Source: CAD feature listing. Evaluate the final solid. Frame: model axes, mm. Round coordinates to 2 decimals unless told otherwise and drop trailing zeros. Order: outer loops, then holes, each group sorted by start corner. A loop starts at its lowest first (then second) coordinate and runs counter-clockwise, first axis right, second up. Notation, with made-up numbers: (-35, 43) -> (4, 43) arc R8 ccw to (4, 57) -> close; hole circle Ø1 at (-19, -17.75). An arc over 180 degrees is marked (long way). Write item = value, one per line. Start each with the question number.
(1) Cut plane A-A on x = 14. Return the cut outline in (y, z) (3 decimals).
(2) Contact query for flat-ended pins moving along their axis: pin 1 Ø2 at (y, z) = (-6, -2.5) entering from +X; pin 2 Ø12 at (y, z) = (-13.5, 16.5) entering from +X; pin 3 Ø3 at (x, y) = (1.5, -11.5) entering from -Z. Output: stop coordinate, or through.
(3) Cut plane B-B on z = 19. Return the cut outline in (x, y), then the cut area to 3 significant figures.
(4) Ray query, line 1 (X direction, y = -10, z = 0); line 2 (Z direction, x = -9.5, y = -7); line 3 (Z direction, x = 12, y = -32). Return the intervals inside material, ascending.
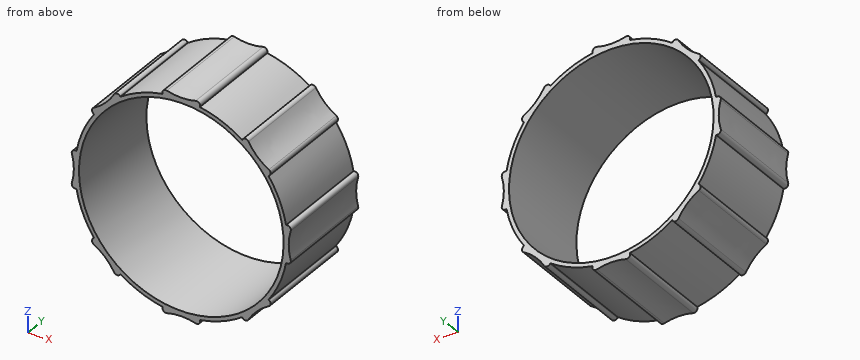
from build123d import *

# Parameters (mm, degrees)
SKETCH3_R           = 37.8587
BOSS_EXTRUDE1_DEPTH = 37.5666


with BuildPart() as part:
    # Sketch3 → Boss-Extrude1 (new body)
    with BuildSketch(Plane(origin=(0, -37.5666, 0), x_dir=(1, 0, 0), z_dir=(0, 1, 0))):
        with BuildLine():
            Line((22.710713351, 32.518210948), (22.542535263, 32.277406051))
            ThreePointArc((22.542535263, 32.277406051), (15.06624702, 36.373135768), (6.883594535, 38.763551242))
            Line((6.883594535, 38.763551242), (6.934949387, 39.052745559))
            ThreePointArc((6.934949387, 39.052745559), (6.539953295, 40.213477214), (5.347634612, 40.499302411))
            add(Edge.make_bspline(
                [(5.347634612, 40.499302411), (0, 39.028097589), (-5.347634612, 40.499302411)],
                knots=[0.133971893, 0.133971893, 0.133971893, 0.866028107, 0.866028107, 0.866028107], degree=2))
            ThreePointArc((-5.347634612, 40.499302411), (-6.539953295, 40.213477214), (-6.934949387, 39.052745559))
            Line((-6.934949387, 39.052745559), (-6.883594478, 38.763550918))
            ThreePointArc((-6.883594478, 38.763550918), (-15.06624685, 36.373135059), (-22.542534901, 32.277404991))
            Line((-22.542534901, 32.277404991), (-22.7107128, 32.518209618))
            ThreePointArc((-22.7107128, 32.518209618), (-23.810778439, 33.059666427), (-24.855984001, 32.418678735))
            add(Edge.make_bspline(
                [(-24.855984001, 32.418678735), (-27.597033743, 27.597031182), (-32.418681395, 24.855981341)],
                knots=[0.133971893, 0.133971893, 0.133971893, 0.866028107, 0.866028107, 0.866028107], degree=2))
            ThreePointArc((-32.418681395, 24.855981341), (-33.059669087, 23.810775779), (-32.518212278, 22.71071014))
            Line((-32.518212278, 22.71071014), (-32.277407381, 22.542532053))
            ThreePointArc((-32.277407381, 22.542532053), (-36.373137098, 15.066243809), (-38.763552571, 6.883591325))
            Line((-38.763552571, 6.883591325), (-39.052746889, 6.934946176))
            ThreePointArc((-39.052746889, 6.934946176), (-40.213478544, 6.539950084), (-40.499303741, 5.347631401))
            add(Edge.make_bspline(
                [(-40.499303741, 5.347631401), (-39.028096259, -3.092e-06), (-40.499303741, -5.347637823)],
                knots=[0.133971893, 0.133971893, 0.133971893, 0.866028107, 0.866028107, 0.866028107], degree=2))
            ThreePointArc((-40.499303741, -5.347637823), (-40.213478544, -6.539956506), (-39.052746889, -6.934952598))
            Line((-39.052746889, -6.934952598), (-38.763552248, -6.883597689))
            ThreePointArc((-38.763552248, -6.883597689), (-36.373136389, -15.066250061), (-32.277406321, -22.542538112))
            Line((-32.277406321, -22.542538112), (-32.518210948, -22.710716011))
            ThreePointArc((-32.518210948, -22.710716011), (-33.059667757, -23.81078165), (-32.418680065, -24.855987212))
            add(Edge.make_bspline(
                [(-32.418680065, -24.855987212), (-27.597028006, -27.597032378), (-24.855982671, -32.418684606)],
                knots=[0.133971893, 0.133971893, 0.133971893, 0.866028107, 0.866028107, 0.866028107], degree=2))
            ThreePointArc((-24.855982671, -32.418684606), (-23.810777109, -33.059672297), (-22.71071147, -32.518215489))
            Line((-22.71071147, -32.518215489), (-22.542533383, -32.277410592))
            ThreePointArc((-22.542533383, -32.277410592), (-15.066245139, -36.373140308), (-6.883592655, -38.763555782))
            Line((-6.883592655, -38.763555782), (-6.934947506, -39.0527501))
            ThreePointArc((-6.934947506, -39.0527501), (-6.539951414, -40.213481755), (-5.347632731, -40.499306952))
            add(Edge.make_bspline(
                [(-5.347632731, -40.499306952), (1.811e-06, -39.028093048), (5.347636493, -40.499306952)],
                knots=[0.133971893, 0.133971893, 0.133971893, 0.866028107, 0.866028107, 0.866028107], degree=2))
            ThreePointArc((5.347636493, -40.499306952), (6.539955176, -40.213481755), (6.934951268, -39.0527501))
            Line((6.934951268, -39.0527501), (6.883596359, -38.763555459))
            ThreePointArc((6.883596359, -38.763555459), (15.066248731, -36.3731396), (22.542536782, -32.277409531))
            Line((22.542536782, -32.277409531), (22.710714681, -32.518214159))
            ThreePointArc((22.710714681, -32.518214159), (23.81078032, -33.059670967), (24.855985882, -32.418683276))
            add(Edge.make_bspline(
                [(24.855985882, -32.418683276), (27.597029251, -27.597029251), (32.418683276, -24.855985882)],
                knots=[0.133971893, 0.133971893, 0.133971893, 0.866028107, 0.866028107, 0.866028107], degree=2))
            ThreePointArc((32.418683276, -24.855985882), (33.059670967, -23.81078032), (32.518214159, -22.710714681))
            Line((32.518214159, -22.710714681), (32.277409262, -22.542536593))
            ThreePointArc((32.277409262, -22.542536593), (36.373138978, -15.06624835), (38.763554452, -6.883595865))
            Line((38.763554452, -6.883595865), (39.05274877, -6.934950717))
            ThreePointArc((39.05274877, -6.934950717), (40.213480425, -6.539954625), (40.499305622, -5.347635942))
            add(Edge.make_bspline(
                [(40.499305622, -5.347635942), (39.028094378, -1.281e-06), (40.499305622, 5.347633282)],
                knots=[0.133971893, 0.133971893, 0.133971893, 0.866028107, 0.866028107, 0.866028107], degree=2))
            ThreePointArc((40.499305622, 5.347633282), (40.213480425, 6.539951965), (39.05274877, 6.934948057))
            Line((39.05274877, 6.934948057), (38.763554129, 6.883593148))
            ThreePointArc((38.763554129, 6.883593148), (36.37313827, 15.06624552), (32.277408202, 22.542533571))
            Line((32.277408202, 22.542533571), (32.518212829, 22.71071147))
            ThreePointArc((32.518212829, 22.71071147), (33.059669637, 23.810777109), (32.418681946, 24.855982671))
            add(Edge.make_bspline(
                [(32.418681946, 24.855982671), (27.597032427, 27.597030616), (24.855984552, 32.418680065)],
                knots=[0.133971893, 0.133971893, 0.133971893, 0.866028107, 0.866028107, 0.866028107], degree=2))
            ThreePointArc((24.855984552, 32.418680065), (23.81077899, 33.059667757), (22.710713351, 32.518210948))
        make_face()
        with Locations(Location((0, 0, 0), (0, 0, 270))):
            Circle(SKETCH3_R, mode=Mode.SUBTRACT)
    extrude(amount=BOSS_EXTRUDE1_DEPTH)


solid = part.part
Evaluation:
q1.outline = (-37.567, -36.797) -> (0, -36.797) -> (0, -35.175) -> (-37.567, -35.175) -> close; (-37.567, 35.175) -> (0, 35.175) -> (0, 36.797) -> (-37.567, 36.797) -> close
q2.pin_1 = 40.08
q2.pin_2 = 37.94
q2.pin_3 = -40
q3.outline = (-34.48, -37.57) -> (-32.75, -37.57) -> (-32.75, 0) -> (-34.48, 0) -> close; (32.75, -37.57) -> (34.48, -37.57) -> (34.48, 0) -> (32.75, 0) -> close
q3.area = 130 mm^2
q4.line_1 = -39.76 to -37.86, 37.86 to 39.76
q4.line_2 = -38.21 to -36.65, 36.65 to 38.21
q4.line_3 = -37.5 to -35.91, 35.91 to 37.5
